```python
from build123d import *

# Parameters (mm, degrees)
BASE_FLANGE1_DEPTH  = 2.5
SKETCH6_W           = 15
SKETCH6_H           = 2.5
BOSS_EXTRUDE1_DEPTH = 15


# Sheet-metal steps are written as plain solids
with BuildPart() as part:
    # Sketch1 → Base-Flange1 (new body)
    with BuildSketch(Plane.XY):
        Polygon((-35, 0), (35, 0), (35, -43), (20, -43), (20, -15), (-31, -15), (-31, -20), (-20, -20), (-20, -43), (-35, -43), align=None)
    extrude(amount=-BASE_FLANGE1_DEPTH)

    # Sketch6 → Boss-Extrude1 (add)
    with BuildSketch(Plane.XY):
        with Locations((-27.5, -41.75)):
            Rectangle(SKETCH6_W, SKETCH6_H)
    boss_extrude1 = extrude(amount=BOSS_EXTRUDE1_DEPTH)

    # Mirror1: Boss-Extrude1 across plane
    add(boss_extrude1.mirror(Plane(origin=(0, 0, 0), x_dir=(0, 0, 1), z_dir=(1, 0, 0))))


solid = part.part
```
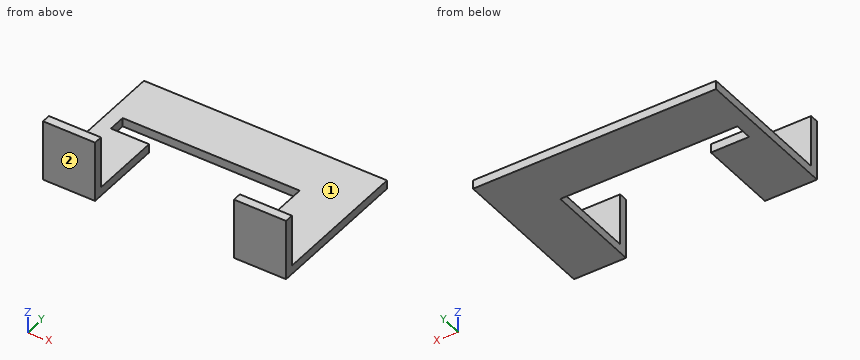
Input: part model. Units: mm. Frame: model coordinates. Face numbers are marked on the shaded views. A direction names the side the tool comes from. Round coordinates to 2 decimals unless told otherwise and drop trailing zeros. Loops run counter-clockwise (first coordinate to the right, second up) from the corner with the lowest first, then second, coordinate; pieces in that order, holes last. Notation, with made-up numbers: (3.5, -14.75) -> (58.5, -14.75) arc R21 ccw to (58.5, 16.25) -> close; hole circle Ø9 at (58.25, -12.5). An arc over 180 degrees is marked (long way). One line per item, written item: value.
(1) Section C-C (x = -26). Return the cut outline in (y, z).
Geometry check:
outline: (-43, -2.5) -> (-20, -2.5) -> (-20, 0) -> (-40.5, 0) -> (-40.5, 15) -> (-43, 15) -> close; (-15, -2.5) -> (0, -2.5) -> (0, 0) -> (-15, 0) -> close
(2) Pin query (flat end, axial travel): pin 1 (2 mm diameter, centred on x = -17.5, z = -1, fed in from -Y); pin 2 (7.5 mm diameter, centred on x = 27.5, z = 6.5, fed in from +Y). Return the tip coordinate at first contact, or that it passes through.
Geometry check:
pin 1: y = -15
pin 2: y = -40.5
(3) Material intervals for line 1 (Y direction, x = -29, z = -0.5); line 2 (Z direction, x = -27, y = -37); line 3 (Y direction, x = 28, z = 12), sorted ascending. Write a range as [from, to].
Geometry check:
line 1: [-43, -20], [-15, 0]
line 2: [-2.5, 0]
line 3: [-43, -40.5]
(4) Section D-D (z = -0.75). Return the cut outline in (x, y).
Geometry check:
outline: (-35, -43) -> (-20, -43) -> (-20, -20) -> (-31, -20) -> (-31, -15) -> (20, -15) -> (20, -43) -> (35, -43) -> (35, 0) -> (-35, 0) -> close
(5) Set-up query: the marked faces 1 and 2. Return all of +Z, -Z, +X, -X, +Y, -Y with unobstructed straight access to the full face (end or side cutting, diameter ignored); none if empty.
Geometry check:
face 1: +Z, +X, -X, +Y
face 2: +Z, -Z, +X, -X, -Y
(6) Section A-A (z = 8.75). Return the cut outline in (x, y), plus the area to 3 significant figures.
Geometry check:
outline: (-35, -43) -> (-20, -43) -> (-20, -40.5) -> (-35, -40.5) -> close; (20, -43) -> (35, -43) -> (35, -40.5) -> (20, -40.5) -> close
area: 75.0 mm2
(7) Section B-B (y = -32). Return the cut outline in (x, z).
Geometry check:
outline: (-35, -2.5) -> (-20, -2.5) -> (-20, 0) -> (-35, 0) -> close; (20, -2.5) -> (35, -2.5) -> (35, 0) -> (20, 0) -> close
